```python
from build123d import *

# Parameters (mm, degrees)
SKETCH1_W               = 10
SKETCH1_H               = 10
BOSS_EXTRUDE1_DEPTH     = 5
CUT_EXTRUDE1_DEPTH      = 9.660254038
CUT_EXTRUDE1_DEPTH_BACK = 9.660254038
SKETCH2_R               = 1.675
SKETCH3_R               = 1.675
CUT_EXTRUDE3_DEPTH      = 2.3
SKETCH4_W               = 10
SKETCH4_H               = 10
BOSS_EXTRUDE2_DEPTH     = 2.7
SKETCH6_W               = 10
SKETCH6_H               = 10
BOSS_EXTRUDE3_DEPTH     = 7
SKETCH9_R               = 2.15
CUT_EXTRUDE12_DEPTH     = 19.468622038
SKETCH10_R              = 1.675
CUT_EXTRUDE13_DEPTH     = 13.003749414
BOSS_EXTRUDE4_DEPTH     = 2.3
SKETCH12_W              = 10
SKETCH12_H              = 10
BOSS_EXTRUDE5_DEPTH     = 2.7
CUT_EXTRUDE14_START     = -2.7
SKETCH13_R              = 1.675
CUT_EXTRUDE14_DEPTH     = 2.7
SKETCH14_R              = 2.15
BOSS_EXTRUDE6_DEPTH     = 0.76
SKETCH16_W              = 10
SKETCH16_H              = 19.7
CUT_EXTRUDE15_DEPTH     = 2.29
BOSS_EXTRUDE7_START     = 1
SKETCH17_W              = 10
SKETCH17_H              = 7.71
SKETCH17_R              = 1.675
BOSS_EXTRUDE7_DEPTH     = 1
SKETCH18_W              = 10
SKETCH18_H              = 7.71
SKETCH18_R              = 1.675
BOSS_EXTRUDE9_DEPTH     = 1
BOSS_EXTRUDE13_DEPTH    = 2.3
SKETCH23_W              = 10
SKETCH23_H              = 10
SKETCH23_R              = 1.675
BOSS_EXTRUDE15_DEPTH    = 2


with BuildPart() as part:
    # Sketch1 → Boss-Extrude1 (new body)
    with BuildSketch(Plane(origin=(0, 0, 0), x_dir=(1, 0, 0), z_dir=(0, 1, 0))):
        Rectangle(SKETCH1_W, SKETCH1_H)
    extrude(amount=BOSS_EXTRUDE1_DEPTH)

    # Sketch2 → Cut-Extrude1 (cut, two sides: drawn at the far end of the back side and taken through both)
    with BuildSketch(Plane(origin=(0, 5, 0), x_dir=(1, 0, 0), z_dir=(0, 1, 0)).offset(-CUT_EXTRUDE1_DEPTH_BACK)):
        with Locations(Location((0, 0, 0), (0, 0, 270))):
            Circle(SKETCH2_R)
    extrude(amount=CUT_EXTRUDE1_DEPTH + CUT_EXTRUDE1_DEPTH_BACK, mode=Mode.SUBTRACT)

    # Sketch3 → Cut-Extrude3 (cut)
    # profile 1 of 2: a face of its own
    with BuildSketch(Plane(origin=(0, 5, 0), x_dir=(1, 0, 0), z_dir=(0, 1, 0))):
        Polygon((-1.56461923, -2.71), (1.56461923, -2.71), (3.129238459, 0), (1.56461923, 2.71), (-1.56461923, 2.71), (-3.129238459, 0), align=None)
        with Locations(Location((0, 0, 0), (0, 0, 270))):
            Circle(SKETCH3_R, mode=Mode.SUBTRACT)
    # profile 2 of 2: a face of its own
    with BuildSketch(Plane(origin=(0, 5, 0), x_dir=(1, 0, 0), z_dir=(0, 1, 0))):
        Polygon((-1.56461923, -2.71), (-3.129238459, 0), (-3.129238459, -5), (3.129238459, -5), (3.129238459, 0), (1.56461923, -2.71), align=None)
    extrude(amount=-CUT_EXTRUDE3_DEPTH, mode=Mode.SUBTRACT)

    # Sketch4 → Boss-Extrude2 (add)
    with BuildSketch(Plane(origin=(0, 5, 0), x_dir=(1, 0, 0), z_dir=(0, 1, 0))):
        Rectangle(SKETCH4_W, SKETCH4_H)
    extrude(amount=BOSS_EXTRUDE2_DEPTH)

    # Sketch6 → Boss-Extrude3 (add)
    with BuildSketch(Plane(origin=(0, 7.7, 0), x_dir=(1, 0, 0), z_dir=(0, 1, 0))):
        Rectangle(SKETCH6_W, SKETCH6_H)
    extrude(amount=BOSS_EXTRUDE3_DEPTH)

    # Sketch9 → Cut-Extrude12 (cut, through all)
    with BuildSketch(Plane(origin=(0, 0, -5), x_dir=(-1, 0, 0), z_dir=(0, 0, -1))):
        with Locations((0, 9.85)):
            Circle(SKETCH9_R)
    extrude(amount=-CUT_EXTRUDE12_DEPTH, mode=Mode.SUBTRACT)

    # Sketch10 → Cut-Extrude13 (cut, through all)
    with BuildSketch(Plane.XZ.offset(-5)):
        with Locations(Location((0, 0, 0), (0, 0, 90))):
            Circle(SKETCH10_R)
    extrude(amount=-CUT_EXTRUDE13_DEPTH, mode=Mode.SUBTRACT)

    # Sketch11 → Boss-Extrude4 (add)
    with BuildSketch(Plane(origin=(0, 14.7, 0), x_dir=(1, 0, 0), z_dir=(0, 1, 0))):
        Polygon((1.56461923, 2.71), (3.129238459, 0), (3.129238459, -5), (5, -5), (5, 5), (-5, 5), (-5, -5), (-3.129238459, -5), (-3.129238459, 0), (-1.56461923, 2.71), align=None)
    extrude(amount=BOSS_EXTRUDE4_DEPTH)

    # Sketch12 → Boss-Extrude5 (add)
    with BuildSketch(Plane(origin=(0, 17, 0), x_dir=(1, 0, 0), z_dir=(0, 1, 0))):
        Rectangle(SKETCH12_W, SKETCH12_H)
    extrude(amount=BOSS_EXTRUDE5_DEPTH)

    # Sketch13 → Cut-Extrude14 (cut)
    with BuildSketch(Plane(origin=(0, 19.7, 0), x_dir=(1, 0, 0), z_dir=(0, 1, 0)).offset(CUT_EXTRUDE14_START)):
        with Locations(Location((0, 0, 0), (0, 0, 270))):
            Circle(SKETCH13_R)
    extrude(amount=CUT_EXTRUDE14_DEPTH, mode=Mode.SUBTRACT)

    # Sketch16 → Cut-Extrude15 (cut)
    with BuildSketch(Plane.XY.offset(5)):
        with Locations((0, 9.85)):
            Rectangle(SKETCH16_W, SKETCH16_H)
    extrude(amount=-CUT_EXTRUDE15_DEPTH, mode=Mode.SUBTRACT)

    # Sketch17 → Boss-Extrude7 (add)
    with BuildSketch(Plane(origin=(0, 0, 0), x_dir=(-1, 0, 0), z_dir=(0, -1, 0)).offset(BOSS_EXTRUDE7_START)):
        with Locations((0, 1.145)):
            Rectangle(SKETCH17_W, SKETCH17_H)
        with Locations(Location((0, 0, 0), (0, 0, 270))):
            Circle(SKETCH17_R, mode=Mode.SUBTRACT)
    extrude(amount=-BOSS_EXTRUDE7_DEPTH)

    # Sketch18 → Boss-Extrude9 (add)
    with BuildSketch(Plane(origin=(0, 19.7, 0), x_dir=(1, 0, 0), z_dir=(0, 1, 0))):
        with Locations((0, 1.145)):
            Rectangle(SKETCH18_W, SKETCH18_H)
        with Locations(Location((0, 0, 0), (0, 0, 270))):
            Circle(SKETCH18_R, mode=Mode.SUBTRACT)
    extrude(amount=BOSS_EXTRUDE9_DEPTH)


with BuildPart() as body_2:
    # Sketch14 → Boss-Extrude6 (new body)
    with BuildSketch(Plane(origin=(0, 0, -5), x_dir=(-1, 0, 0), z_dir=(0, 0, -1))):
        with Locations((0, 9.85)):
            Circle(SKETCH14_R)
    extrude(amount=-BOSS_EXTRUDE6_DEPTH)


    add(part.part)  # Boss-Extrude13 merges part
    # Sketch22 → Boss-Extrude13 (add)
    with BuildSketch(Plane(origin=(0, 0, -5), x_dir=(-1, 0, 0), z_dir=(0, 0, -1))):
        Polygon((-5, 12.979238459), (0, 12.979238459), (2.71, 11.41461923), (2.71, 8.28538077), (0, 6.720761541), (-5, 6.720761541), (-5, 4.85), (5, 4.85), (5, 14.85), (-5, 14.85), align=None)
    extrude(amount=BOSS_EXTRUDE13_DEPTH)

    # Sketch23 → Boss-Extrude15 (add)
    with BuildSketch(Plane(origin=(0, 0, -7.3), x_dir=(-1, 0, 0), z_dir=(0, 0, -1))):
        with Locations((0, 9.85)):
            Rectangle(SKETCH23_W, SKETCH23_H)
        with Locations((0, 9.85)):
            Circle(SKETCH23_R, mode=Mode.SUBTRACT)
    extrude(amount=BOSS_EXTRUDE15_DEPTH)


solid = body_2.part
```
Could you check a few things on this model? Use its own coordinates, in mm. A direction names the side the tool comes from. Round coordinates to 2 decimals unless told otherwise and drop trailing zeros. Write each loop counter-clockwise with the first axis right and the second up, starting at its lowest first coordinate (ties: lowest second). Pieces come first, ordered by that corner, then holes.
(1) For pin 1 (2.5 mm diameter, centred on x = 0, y = 9.85, fed in from -Z); pin 2 (3 mm diameter, centred on x = 0, z = 0, fed in from -Y); pin 3 (1.2 mm diameter, centred on y = 9.5, z = -6.5, fed in from +X); pin 4 (1.8 mm diameter, centred on x = 3, z = -6, fed in from -Y), each with a flat end and sliding along its axis, tell me the tip position at first contact or that it passes through.
Findings below:
pin 1: stops at z = -5
pin 2: passes through
pin 3: stops at x = -2.71
pin 4: stops at y = 4.85
(2) Suppose I cut it at A-A on y = 6.25. Write out the boundary of the cut face in (x, z) (3 decimals).
Findings below:
outline: (-5, -9.3) - (5, -9.3) - (5, 2.71) - (-5, 2.71) - close; hole circle Ø3.35 at (0, 0)
(3) Suppose I cut it at C-C on y = 9.85. Write out the boundary of the cut face in (x, z) (3 decimals).
Findings below:
outline: (-5, -9.3) - (-1.675, -9.3) - (-1.675, -7.3) - (-2.71, -7.3) - (-2.71, -5) - (5, -5) - (5, 2.71) - (2.15, 2.71) - (2.15, -4.24) - (-2.15, -4.24) - (-2.15, 2.71) - (-5, 2.71) - close; (1.675, -9.3) - (5, -9.3) - (5, -7.3) - (1.675, -7.3) - close
(4) Suppose I cut it at D-D on z = 0.5. Write out the boundary of the cut face in (x, y), and give its area (3 significant figures).
Findings below:
outline: (-5, -1) - (-1.6, -1) - (-1.6, 2.7) - (-3.13, 2.7) - (-3.13, 5) - (-1.6, 5) - (-1.6, 8.41) arc R2.15 cw to (-1.6, 11.29) - (-1.6, 14.7) - (-3.13, 14.7) - (-3.13, 17) - (-1.6, 17) - (-1.6, 20.7) - (-5, 20.7) - close; (1.6, -1) - (5, -1) - (5, 20.7) - (1.6, 20.7) - (1.6, 17) - (3.13, 17) - (3.13, 14.7) - (1.6, 14.7) - (1.6, 11.29) arc R2.15 cw to (1.6, 8.41) - (1.6, 5) - (3.13, 5) - (3.13, 2.7) - (1.6, 2.7) - close
area: 131 mm2
(5) Thinking about a two-plate mould opening in X: for faces 1 (the face through (-1.336, 12.208, -6.134)), 2 (the face through (2.358, 3.866, -1.336)), 3 (the face through (2, 6.721, -6)), which applies, +X half, -X half, draft (parallel to the pull), parting line (faces both ways), or undercut?
Findings below:
face 1: +X half
face 2: undercut
face 3: draft
(6) If I drill on probe 1 along Y at (x, z) = (2, -6.5); probe 2 along Z at (x, y) = (2, 10.5); probe 3 along Y at (x, z) = (1.75, -2), over which ranges is the centre line in solid material (lowest first)?
Findings below:
probe 1: y = 4.85 to 6.72, 12.98 to 14.85
probe 2: z = -9.3 to -7.3, -5 to -4.24
probe 3: y = -1 to 2.7, 5 to 8.6, 11.1 to 14.7, 17 to 20.7
(7) Which directions (+Z, -Z, +X, -X, +Y, -Y) give clear straight access to the entire face, cutting with the end or side of a thin tool? Please do faces 4 (the face through (-1.37, 7.51, -6.13)), 5 (the face through (0, 4.85, -7)), 6 (the face through (-2.358, 15.834, -1.336)).
Findings below:
face 4: +X
face 5: -Z, +X, -X, -Y
face 6: +Z
(8) Suppose I cut it at B-B on z = -6.25. Write out the boundary of the cut face in (x, y), and give its area (3 significant figures).
Findings below:
outline: (-5, 4.85) - (5, 4.85) - (5, 6.72) - (0, 6.72) - (-2.71, 8.29) - (-2.71, 11.41) - (0, 12.98) - (5, 12.98) - (5, 14.85) - (-5, 14.85) - close
area: 56.0 mm2
